```python
from build123d import *

# Parameters (mm, degrees)
EXTRUDE_2_DEPTH              = 280
HOLE_WIZARD_M4_1_D           = 4.5
HOLE_WIZARD_M4_1_CBORE_D     = 8.6
HOLE_WIZARD_M4_1_CBORE_DEPTH = 2.2
HOLE_WIZARD_M4_3_D           = 4.5
HOLE_WIZARD_M4_3_CBORE_D     = 8.6
HOLE_WIZARD_M4_3_CBORE_DEPTH = 2.2


with BuildPart() as part:
    # ｽｹｯﾁ1 → ﾎﾞｽ - 押し出し2 (new body)
    with BuildSketch(Plane.XY):
        Polygon((0, 0), (20, 0), (20, 7.2), (16.2, 7.2), (16.2, 5.969681415), (18.2, 5.969681415), (18.2, 3), (1.8, 3), (1.8, 6), (3.8, 6), (3.8, 7.2), (0, 7.2), align=None)
    extrude(amount=EXTRUDE_2_DEPTH)

    # M4 丸押えねじ用座ぐり穴1 (through all)
    with Locations(Plane(origin=(0, 3, 0), x_dir=(1, 0, 0), z_dir=(0, 1, 0))):
        with Locations((10, -255), (10, -205), (10, -155), (10, -105), (10, -55)):
            CounterBoreHole(HOLE_WIZARD_M4_1_D / 2, HOLE_WIZARD_M4_1_CBORE_D / 2, HOLE_WIZARD_M4_1_CBORE_DEPTH)

    # M4 丸押えねじ用座ぐり穴3 (through all)
    with Locations(Plane(origin=(0, 3, 0), x_dir=(1, 0, 0), z_dir=(0, 1, 0))):
        with Locations((10, -5)):
            CounterBoreHole(HOLE_WIZARD_M4_3_D / 2, HOLE_WIZARD_M4_3_CBORE_D / 2, HOLE_WIZARD_M4_3_CBORE_DEPTH)


solid = part.part
```
Check sheet for the modelled part. Datum: model origin and axes. Units: mm. A direction names the side the tool comes from. Coordinates: 2 decimals unless noted, no trailing zeros. Order: outer loops, then holes, each group sorted by start corner. A loop starts at its lowest first (then second) coordinate and runs counter-clockwise, first axis right, second up. Notation, with made-up numbers: M 71,27.25 L 123,27.25 A19 cw 123,51.25 Z; hole C -19,80.25 d8. An arc over 180 degrees is marked long. One line per question, with ' | ' between items. Start each with the question number.
Item 1: Gauge pin test, flat ends, axial feed: P1, Ø1, axis at x = 14, z = 108.5, coming from the +Y side; P2, Ø2.5, axis at x = 8.5, z = 254.5, coming from the +Y side. Record the tip position at first contact, or that the pin passes through.
Item 2: Sectioned sample at B-B on z = 169.5. Record the cut outline in (x, y), and give its area (3 significant figures).
Item 3: Mould release check, pull along Z, two halves, no side actions. Record for faces 1 (the flat face through (10, 2, 0)), 2 (the flat face through (10, 0, 138)), 3 (the cylindrical face through (10.29, 0.39, 252.77)), 4 (the flat face through (10, 2, 280)): pulls with the +Z half, pulls with the -Z half, needs draft (parallel to the pull), parting line crosses it, or undercut.
Item 4: Access from +Z, -Z, +X, -X, +Y, -Y to the whole of each face (thin tool, end or side, straight path). Record for faces 5 (the flat face through (10, 3, 138)), 6 (the cylindrical face through (10.488, 0.394, 157.196)), 7 (the flat face through (12, 0.8, 7)).
Item 5: Material ranges on line 1 (Y direction, x = 3.75, z = 208); line 2 (X direction, y = 0.4, z = 205); line 3 (X direction, y = 1.45, z = 255), recorded low to high.
Item 6: Sectioned sample at A-A on z = 5. Record the cut outline in (x, y), and give its area (3 significant figures).
Answer below:
1) P1: stops at y = 3 | P2: stops at y = 0.8
2) outline: M 0,0 L 20,0 L 20,7.2 L 16.2,7.2 L 16.2,5.97 L 18.2,5.97 L 18.2,3 L 1.8,3 L 1.8,6 L 3.8,6 L 3.8,7.2 L 0,7.2 Z | area: 80.0 mm^2
3) face 1: pulls with the -Z half | face 2: needs draft | face 3: undercut | face 4: pulls with the +Z half
4) face 5: +Z, -Z | face 6: +Y, -Y | face 7: +Y
5) line 1: y = 0 to 3, 6 to 7.2 | line 2: x = 0 to 7.75, 12.25 to 20 | line 3: x = 0 to 5.7, 14.3 to 20
6) outline: M 0,0 L 7.75,0 L 7.75,0.8 L 5.7,0.8 L 5.7,3 L 1.8,3 L 1.8,6 L 3.8,6 L 3.8,7.2 L 0,7.2 Z; M 12.25,0 L 20,0 L 20,7.2 L 16.2,7.2 L 16.2,5.97 L 18.2,5.97 L 18.2,3 L 14.3,3 L 14.3,0.8 L 12.25,0.8 Z | area: 57.5 mm^2
